Autodesk Inventor part; units mm, degrees
ref_plane "YZ Plane" through (0, 0, 0) normal (1, 0, 0) x (0, 1, 0)
ref_plane "XZ Plane" through (0, 0, 0) normal (0, 1, 0) x (-1, 0, 0)
ref_plane "XY Plane" through (0, 0, 0) normal (0, 0, 1) x (1, 0, 0)
sketch "Sketch1" plane through (0, 0, 0) normal (0, 1, 0) x (-1, 0, 0)
  line L0 (0, 0) -> (50.8, 0)
  line L1 (50.8, 0) -> (50.8, -736.6)
  line L2 (50.8, -736.6) -> (0, -736.6)
  line L3 (0, -736.6) -> (0, 0)
  dimension "d0" = 50.8
  dimension "d1" = 736.6
extrude "Extrusion1" add sketch "Sketch1" along normal blind 6.35
sketch "Sketch2" plane through (0, 6.35, 0) normal (0, 1, 0) x (1, 0, 0)
  line L0 (-50.8, 0) -> (-44.45, 0)
  line L1 (-50.8, 0) -> (0, 0)
  line L2 (-44.45, 0) -> (-44.45, 736.6)
  line L3 (0, 736.6) -> (-50.8, 736.6)
  line L4 (-44.45, 736.6) -> (-50.8, 736.6)
  line L5 (-50.8, 736.6) -> (-50.8, 0)
  line L6 (-50.8, 0) -> (-44.45, 0)
  dimension "d4" = 6.35
  dimension "d5" = 736.6
  dimension "d6" = 736.6
extrude "Extrusion2" add sketch "Sketch2" along normal blind 44.45
fillet "Fillet1" radius 6.35 1 edges at (-44.45, 6.35, -368.3)
fillet "Fillet2" radius 6.35 1 edges at (0, 6.35, -368.3)
fillet "Fillet3" radius 6.35 1 edges at (-44.45, 50.8, -368.3)
hole "Hole1" at (-44.45, 25.4, -184.15) direction (-1, 0, 0) diameter 14.605 end through all
pattern_linear "Rectangular Pattern1" count 3 spacing 152.4 along (0, 0, -1) of "Hole1"
sketch "Sketch4" plane through (-44.45, 12.7, 0) normal (1, 0, 0) x (0, 0, -1)
  line L0 (43.5102, 15.9813) -> (43.5102, 68.613)
  line L1 (43.5102, 68.613) -> (43.5102, -117.0764)
  line L2 (43.5102, -117.0764) -> (-179.7757, -29.554)
  line L3 (-179.7757, -29.554) -> (-128.9181, 50.2806)
  line L4 (-128.9181, 50.2806) -> (-52.0403, 93.4505)
  line L5 (-52.0403, 93.4505) -> (43.5102, 68.613)
  point P0 (0, -12.7)
extrude "Extrusion3" cut sketch "Sketch4" along normal through all both and the other way through all
sketch "Sketch6" plane through (-50.8, 0, -736.6) normal (-1, 0, 0) x (0, 0, 1)
  line L0 (0, 0) -> (31.75, 0)
  line L1 (693.0898, 0) -> (0, 0)
  line L2 (31.75, 0) -> (31.75, 50.8)
  line L3 (0, 50.8) -> (693.0898, 50.8)
  line L4 (0, 0) -> (0, 19.05)
  line L5 (0, 0) -> (0, 50.8)
  line L6 (0, 19.05) -> (31.75, 50.8)
  line L7 (31.75, 87.3968) -> (-26.0736, 76.8736)
  line L8 (-26.0736, 76.8736) -> (-32.5199, 38.9128)
  line L9 (-32.5199, 38.9128) -> (0, 19.05)
  line L10 (31.75, 87.3968) -> (31.75, 50.8)
  point P0 (736.6, 0)
  dimension "d38" = 31.75
  dimension "d39" = 19.05
extrude "Extrusion4" cut sketch "Sketch6" against normal blind 304.8 contours L5 L3 L6
sketch "Sketch7" plane through (-50.8, 0, -736.6) normal (-1, 0, 0) x (0, 0, 1)
  line L0 (0, 0) -> (0, 6.35)
  line L1 (0, 0) -> (0, 19.05)
  line L2 (0, 6.35) -> (0, 61.7609)
  line L3 (0, 61.7609) -> (31.75, 50.8)
  line L4 (31.75, 50.8) -> (57.15, 50.8)
  line L5 (31.75, 50.8) -> (693.0898, 50.8)
  line L6 (57.15, 50.8) -> (0, 6.35)
  point P0 (736.6, 0)
  dimension "d42" = 6.35
  dimension "d43" = 25.4
extrude "Extrusion5" cut sketch "Sketch7" against normal blind 304.8
sketch "Sketch10" plane through (0, 6.35, 0) normal (0, 1, 0) x (1, 0, 0)
  circle A0 centre (-10.8427, 725.424) radius 2.667
  circle A1 centre (-33.7027, 727.71) radius 2.667
  point P0 (0, 0)
extrude "Extrusion6" cut sketch "Sketch10" against normal blind 25.4
sketch "Sketch12" plane through (-50.8, 0, -736.6) normal (-1, 0, 0) x (0, 0, 1)
  circle A0 centre (400.05, 25.4) radius 7.3025
  circle A1 centre (552.45, 25.4) radius 7.3025
  circle A2 centre (247.65, 25.4) radius 7.3025
  circle A3 centre (247.65, 25.4) radius 14.2875
  circle A4 centre (400.05, 25.4) radius 14.2875
  circle A5 centre (552.45, 25.4) radius 14.2875
  point P0 (736.6, 0)
  dimension "d48" = 28.575
  dimension "d49" = 28.575
  dimension "d50" = 28.575
extrude "Extrusion7" cut sketch "Sketch12" against normal blind 25.4
sketch "Sketch13" plane through (0, 6.35, 0) normal (0, 1, 0) x (1, 0, 0)
  circle A0 centre (-25.4, 68.2719) radius 3.175
  circle A1 centre (-25.4, 104.4702) radius 3.175
  point P0 (0, 0)
extrude "Extrusion8" cut sketch "Sketch13" against normal blind 25.4
sketch "Sketch14" plane through (0, 6.35, 0) normal (0, 1, 0) x (1, 0, 0)
  circle A0 centre (-25.4, 68.2719) radius 3.175
  circle A1 centre (-25.4, 104.4702) radius 3.175
  circle A2 centre (-10.8427, 725.424) radius 2.667
  circle A3 centre (-33.7027, 727.71) radius 2.667
  line L0 (-38.1, 43.5102) -> (-6.35, 43.5102)
  line L1 (-6.35, 736.6) -> (-6.35, 43.5102)
  line L2 (-6.35, 736.6) -> (-38.1, 736.6)
  line L3 (-38.1, 43.5102) -> (-38.1, 736.6)
  line L4 (-6.35, 43.5102) -> (0, 43.5102)
  line L5 (0, 736.6) -> (0, 43.5102)
  line L6 (0, 736.6) -> (-6.35, 736.6)
  line L7 (-6.35, 736.6) -> (-6.35, 43.5102)
  line L8 (11.781, 501.9003) -> (-12.6385, 502.7611)
  line L9 (-13.1288, 510.961) -> (-13.1288, 506.3701)
  line L10 (-13.1288, 503.6795) -> (-13.1288, 506.3701)
  ellipse E0 centre (-12.6208, 503.2688) end of major axis (-12.1128, 503.2688) minor radius 0.508 (-13.1288, 503.2688) -> (-12.6385, 502.7611) ccw
  line L11 (-13.1288, 518.5072) -> (-13.1288, 510.961)
  line L12 (-13.1288, 526.3619) -> (-13.1288, 520.4519)
  line L13 (-13.1288, 518.5844) -> (-13.1288, 520.4519)
  line L14 (-21.3838, 525.728) -> (-6.0168, 525.728)
  line L15 (-21.3838, 530.5032) -> (-21.3838, 525.728)
  line L16 (-21.3838, 530.5032) -> (-6.0168, 530.5032)
  line L17 (-13.9225, 584.3659) -> (-13.9225, 520.3579)
  line L18 (-15.6688, 579.6293) -> (-15.6688, 550.0287)
  line L19 (-21.8918, 577.0337) -> (-21.8918, 580.7929)
  line L20 (-15.6688, 589.4756) -> (-15.6688, 583.2973)
  line L21 (-14.1739, 593.5184) -> (5.7789, 610.1541)
  line L22 (-13.4799, 597.3719) -> (6.1422, 615.7328)
  line L23 (0, 736.6) -> (0, 43.5102)
  line L24 (0, 482.6) -> (-28.575, 482.6)
  line L25 (-28.575, 482.6) -> (-28.575, 622.3)
  line L26 (-28.575, 622.3) -> (0, 622.3)
  line L27 (0, 622.3) -> (0, 482.6)
  point P0 (0, 0)
  dimension "d55" = 139.7
extrude "Extrusion9" cut sketch "Sketch14" against normal blind 6.35 contours L24 L25 L26 L1 L16 L15 L14 | L1 L8 L5 L24 | L1 L21 L5 L8 | L26 L5 L22 L1 | L14 L17 L16 L1 | L22 L5 L21 L1 | L17 L14 L15 L16
properties part number "2x2 quarter in angle aluminum far side"
Geometry check sheet. Reference: the model listing, model coordinates, mm. A direction names the side the tool comes from. Round coordinates to 2 decimals unless told otherwise and drop trailing zeros. Loops run counter-clockwise (first coordinate to the right, second up) from the corner with the lowest first, then second, coordinate; pieces in that order, holes last. Notation, with made-up numbers: (-27, 85.5) -> (8, 85.5) arc R23 ccw to (8, 111.5) -> close; hole circle Ø8 at (48, 14). An arc over 180 degrees is marked (long way). Answer as a JSON object with one key per item and string values. Group by question number.
Item 1: Set-up check for faces 5 (the face through (-44.45, 28, -381)), 6 (the face through (-50.8, 25, -385)): record each of +Z, -Z, +X, -X, +Y, -Y from which the full face is reachable in a straight line by a thin tool's end or side.
Item 2: Release check for a two-part mould opening along Z. For faces 1 (the face through (-25, 0, -385)), 2 (the face through (-47.57, 19.93, -170.95)), 3 (the face through (-47.36, 28.89, -707.62)), 4 (the face through (-47.57, 26.028, -350.824)) record: pulls with the +Z half, pulls with the -Z half, needs draft (parallel to the pull), parting line crosses it, or undercut.
Item 3: Cross-section at B-B, the plane y = 25.4. Record the cut outline in (x, z).
Item 4: Depth check by flat-ended pin: pin 1 Ø16 at (x, z) = (-28.5, -224.5) entering from +Y; pin 2 Ø23 at (y, z) = (25.4, -184.15) entering from +X; pin 3 Ø8 at (y, z) = (5.5, -138.5) entering from +X; pin 4 Ø9.5 at (y, z) = (34, -534) entering from +X. Enter the tip coordinate at first touch or a pass-through.
Item 5: Thickness scan on line 1 along Z through (x, y) = (-25.4, 3); line 2 along Z through (x, y) = (-48.5, 25.4); line 3 along Z through (x, y) = (-19, 2). Record the ranges inside material, lowest first.
Determined:
{
 "1": {"face 5": "+Z, -Z, +X, +Y", "face 6": "+Z, -Z, -X, +Y, -Y"},
 "2": {"face 1": "needs draft", "face 2": "undercut", "face 3": "pulls with the -Z half", "face 4": "undercut"},
 "3": {"outline": "(-50.8, -712.11) -> (-44.45, -712.11) -> (-44.45, -503.24) -> (-50.8, -503.24) -> close; (-50.8, -474.66) -> (-44.45, -474.66) -> (-44.45, -350.84) -> (-50.8, -350.84) -> close; (-50.8, -322.26) -> (-44.45, -322.26) -> (-44.45, -198.44) -> (-50.8, -198.44) -> close; (-50.8, -169.86) -> (-44.45, -169.86) -> (-44.45, -43.51) -> (-50.8, -43.51) -> close"},
 "4": {"pin 1": "stops at y = 6.35", "pin 2": "passes through", "pin 3": "stops at x = -0.18", "pin 4": "stops at x = -44.45"},
 "5": {"line 1": "z = -736.6 to -622.3, -482.6 to -107.65, -101.3 to -71.45, -65.1 to -43.51", "line 2": "z = -712.11 to -503.24, -474.66 to -350.84, -322.26 to -198.44, -169.86 to -43.51", "line 3": "z = -736.6 to -622.3, -482.6 to -43.51"}
}
